The model under review builds one solid part; all positions refer to its coordinate system, in mm. Face numbers are marked on the shaded views. Round coordinates to 2 decimals unless told otherwise and drop trailing zeros. Order: outer loops, then holes, each group sorted by start corner. A loop starts at its lowest first (then second) coordinate and runs counter-clockwise, first axis right, second up. Notation, with made-up numbers: (33, 0) -> (85, 0) arc R9 ccw to (85, 17) -> close; hole circle Ø6 at (-33, 81). An arc over 180 degrees is marked (long way). Use a Markdown table: item, result. Add a question column.
```python
from build123d import *

# Parameters (mm, degrees)
SKETCH1_W                                         = 241.5
SKETCH1_H                                         = 22
BASE_FLANGE1_DEPTH                                = 2.5
EDGE_FLANGE1_STRIP_W                              = 11.4732
EDGE_FLANGE1_STRIP_H                              = 2.5
EDGE_FLANGE1_STRIP_CUT_DEPTH                      = 220
EDGE_FLANGE1_RELIEF_W                             = 12.7232
EDGE_FLANGE1_RELIEF_H                             = 1.25
EDGE_FLANGE1_RELIEF_CUT_DEPTH                     = 2.5
EDGE_FLANGE1_DEPTH                                = 220
CUT_EXTRUDE1_DEPTH                                = 2.5
CSK_FOR_3_FLAT_HEAD_MACHINE_SCREW_100_D           = 2.794
CSK_FOR_3_FLAT_HEAD_MACHINE_SCREW_100_CSINK_D     = 5.0546
CSK_FOR_3_FLAT_HEAD_MACHINE_SCREW_100_CSINK_ANGLE = 100


# Sheet-metal steps are written as plain solids
with BuildPart() as part:
    # Sketch1 → Base-Flange1 (new body)
    with BuildSketch(Plane.XY):
        with Locations((-120.75, 11)):
            Rectangle(SKETCH1_W, SKETCH1_H)
    extrude(amount=-BASE_FLANGE1_DEPTH)

    # Edge-Flange1 strip (across the edge) → Edge-Flange1 strip cut (cut)
    with BuildSketch(Plane(origin=(-220, 22, -2.5), x_dir=(0, -1, 0), z_dir=(1, 0, 0))):
        with Locations((-2.5, -1.25)):
            Rectangle(EDGE_FLANGE1_STRIP_W, EDGE_FLANGE1_STRIP_H)
    extrude(amount=EDGE_FLANGE1_STRIP_CUT_DEPTH, mode=Mode.SUBTRACT)

    # Edge-Flange1 relief (on the sheet) → Edge-Flange1 relief cut (cut)
    with BuildSketch(Plane(origin=(-220, 18.7634, -2.5), x_dir=(0, -1, 0), z_dir=(0, 0, -1))):
        with Locations((-5.1116, 0.625)):
            Rectangle(EDGE_FLANGE1_RELIEF_W, EDGE_FLANGE1_RELIEF_H)
    extrude(amount=-EDGE_FLANGE1_RELIEF_CUT_DEPTH, mode=Mode.SUBTRACT)

    # Edge-Flange1 section (across the edge) → Edge-Flange1 (add)
    with BuildSketch(Plane(origin=(-220, 22, -2.5), x_dir=(0, -1, 0), z_dir=(1, 0, 0))):
        with BuildLine():
            Line((0, 0.7366), (0, 7.5))
            Line((0, 7.5), (2.5, 7.5))
            Line((2.5, 7.5), (2.5, 0.7366))
            ThreePointArc((2.5, 0.7366), (2.715745145, 0.215745145), (3.2366, 0))
            Line((3.2366, 0), (3.2366, -2.5))
            ThreePointArc((3.2366, -2.5), (0.947978192, -1.552021808), (0, 0.7366))
        make_face()
    extrude(amount=EDGE_FLANGE1_DEPTH)

    # Sketch13 → Cut-Extrude1 (cut)
    with BuildSketch(Plane.XY):
        with BuildLine():
            Line((-235.5, 18.9), (-229.5, 18.9))
            ThreePointArc((-229.5, 18.9), (-226.5, 15.9), (-229.5, 12.9))
            Line((-229.5, 12.9), (-235.5, 12.9))
            ThreePointArc((-235.5, 12.9), (-238.5, 15.9), (-235.5, 18.9))
        make_face()
    extrude(amount=-CUT_EXTRUDE1_DEPTH, mode=Mode.SUBTRACT)

    # CSK for #3 Flat Head Machine Screw (100)1 (through all)
    with Locations(Plane(origin=(0, 22, 0), x_dir=(1, 0, 0), z_dir=(0, 1, 0))):
        with Locations((-213, 7)):
            CounterSinkHole(CSK_FOR_3_FLAT_HEAD_MACHINE_SCREW_100_D / 2, CSK_FOR_3_FLAT_HEAD_MACHINE_SCREW_100_CSINK_D / 2, counter_sink_angle=CSK_FOR_3_FLAT_HEAD_MACHINE_SCREW_100_CSINK_ANGLE)

    # Mirror1: part across plane


with BuildPart() as part_1:
    add(part.part)
    add(part.part.mirror(Plane(origin=(0, 0, -2.5), x_dir=(0, 0, 1), z_dir=(1, 0, 0))))

    # Mirror2: part across face


with BuildPart() as part_2:
    add(part_1.part)
    add(part_1.part.mirror(Plane(origin=(0, 0, -1.25), x_dir=(0, 0, 1), z_dir=(0, -1, 0))))


solid = part_2.part
```
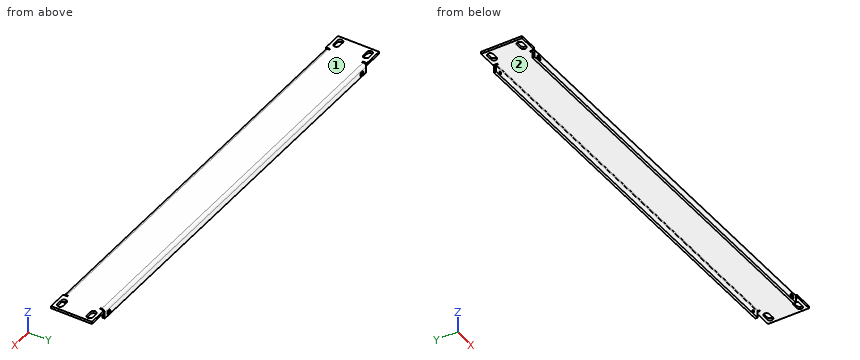
Q1. Add section B-B, the plane y = 0. Give the boundary of the cut face in (x, z).
Q2. Add section A-A, the plane x = 159. Give the boundary of the cut face in (y, z).
Q3. Draft analysis for pull direction Z (two halves, no side actions). For the marked faces 1 and 2, state which applies: released by +Z, released by -Z, zero draft, split by the parting line, or undercut.
Q4. For pin 1 (5 mm diameter, centred on y = -20, z = -6, fed in from -X); pin 2 (3.5 mm diameter, centred on x = 213, z = -7, fed in from -Y); pin 3 (4 mm diameter, centred on y = -9, z = -5, fed in from -X); pin 4 (10 mm diameter, centred on x = -57, y = 11.5, fed in from -Z), all flat-tipped, find the tip position at first contact; note any pin that passes through.
Q5. To check wall thickness, follow line 1 along X through (y, z) = (20.5, -7); line 2 along X through (y, z) = (15.5, -2); line 3 along Y through (x, z) = (35.5, -8.25). State the ranges of each line that lie inside material, in increasing order.
Return value:
| question | item | result |
|---|---|---|
| 1 | outline | (-241.5, -2.5) -> (241.5, -2.5) -> (241.5, 0) -> (-241.5, 0) -> close |
| 2 | outline | (-22, -10) -> (-19.5, -10) -> (-19.5, -3.24) arc R0.74 cw to (-18.76, -2.5) -> (18.76, -2.5) arc R0.74 cw to (19.5, -3.24) -> (19.5, -10) -> (22, -10) -> (22, -3.24) arc R3.24 ccw to (18.76, 0) -> (-18.76, 0) arc R3.24 ccw to (-22, -3.24) -> close |
| 3 | face 1 | released by +Z |
| 3 | face 2 | released by -Z |
| 4 | pin 1 | x = -220 |
| 4 | pin 2 | y = -21.35 |
| 4 | pin 3 | through |
| 4 | pin 4 | z = -2.5 |
| 5 | line 1 | -220 to -214.4, -211.6 to 211.6, 214.4 to 220 |
| 5 | line 2 | -241.5 to -238.47, -226.53 to 226.53, 238.47 to 241.5 |
| 5 | line 3 | -22 to -19.5, 19.5 to 22 |
